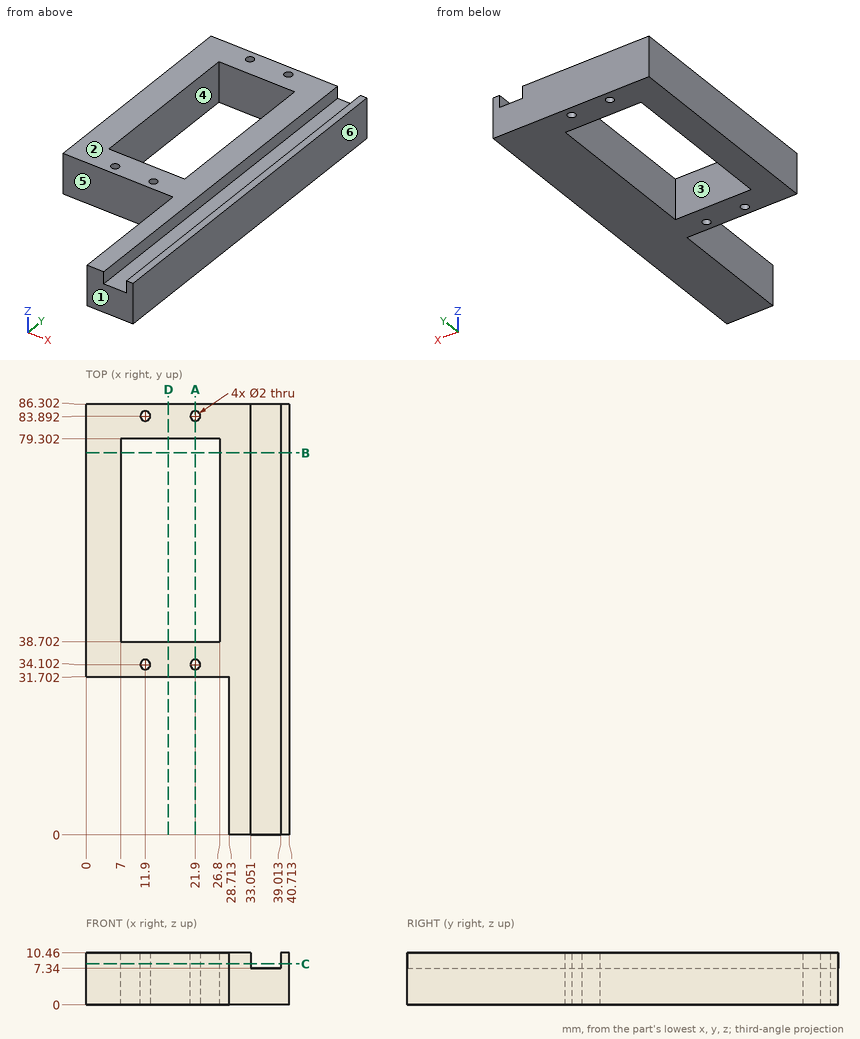
Design review of the part shown in the three views and the two pictorial views. Dimensions are in mm from the part's minimum x, y and z. A direction names the side the tool comes from. Give positions to 0.01 mm unless a question says otherwise; leave off trailing zeros. Loops run counter-clockwise (first coordinate to the right, second up) from the corner with the lowest first, then second, coordinate; pieces in that order, holes last. Notation, with made-up numbers: (34, 62.25) -> (64, 62.25) arc R30 cw to (64, 91.25) -> close; hole circle Ø9 at (51.25, -26.5). An arc over 180 degrees is marked (long way). Answer as a JSON object with one key per item and string values. Group by question number.
Q1. Draft analysis for pull direction Y (two halves, no side actions). For the marked faces 1, 2 and 3, state which applies: pulls with the +Y half, pulls with the -Y half, needs draft (parallel to the pull), parting line crosses it, or undercut.
Q2. Wall thickness on line 1 along Y through (x, z) = (11.9, 4); line 2 along X through (y, z) = (58, 8.75); line 3 along Y through (x, z) = (24, 9.75): over which ranges is each line inside the solid? List them lowest first.
Q3. Tool access review of the marked faces 4, 5 and 6: name each direction out of +Z, -Z, +X, -X, +Y, -Y from which nothing blocks a thin tool from reaching the whole face with its end or side.
Q4. Insertion check: pin 1 (3 mm diameter, centred on x = 21.9, y = 83.89, fed in from -Z); pin 2 (0.9 mm diameter, centred on y = 28, z = 9.5, fed in from -X); pin 3 (1.8 mm diameter, centred on x = 36.5, y = 50.5, fed in from +Z); pin 4 (3 mm diameter, centred on x = 21, z = 2.5, fed in from -Y). Each pin has a flat end and moves straight along its axis. Give the tip position at first contact, or say it passes through.
Q5. Take a section at A-A (x = 21.9). Write out the cut boundary in (y, z).
Q6. Take a section at D-D (x = 16.5). Write out the cut boundary in (y, z), plus the area to 3 significant figures.
Q7. Take a section at B-B (y = 76.5). Write out the cut boundary in (x, z), plus the area to 3 significant figures.
Q8. Take a section at C-C (z = 8.25). Write out the cut boundary in (x, y), plus the area to 3 significant figures.
Answer below:
{
 "1": {"face 1": "pulls with the -Y half", "face 2": "needs draft", "face 3": "undercut"},
 "2": {"line 1": "y = 31.7 to 33.1, 35.1 to 38.7, 79.3 to 82.89, 84.89 to 86.3", "line 2": "x = 0 to 7, 26.8 to 33.05, 39.01 to 40.71", "line 3": "y = 31.7 to 38.7, 79.3 to 86.3"},
 "3": {"face 4": "+Z, -Z", "face 5": "+Z, -Z, -X, -Y", "face 6": "+Z, -Z, +X, +Y, -Y"},
 "4": {"pin 1": "stops at z = 0", "pin 2": "stops at x = 28.71", "pin 3": "stops at z = 7.34", "pin 4": "stops at y = 31.7"},
 "5": {"outline": "(31.7, 0) -> (33.1, 0) -> (33.1, 10.46) -> (31.7, 10.46) -> close; (35.1, 0) -> (38.7, 0) -> (38.7, 10.46) -> (35.1, 10.46) -> close; (79.3, 0) -> (82.89, 0) -> (82.89, 10.46) -> (79.3, 10.46) -> close; (84.89, 0) -> (86.3, 0) -> (86.3, 10.46) -> (84.89, 10.46) -> close"},
 "6": {"outline": "(31.7, 0) -> (38.7, 0) -> (38.7, 10.46) -> (31.7, 10.46) -> close; (79.3, 0) -> (86.3, 0) -> (86.3, 10.46) -> (79.3, 10.46) -> close", "area": "146 mm2"},
 "7": {"outline": "(0, 0) -> (7, 0) -> (7, 10.46) -> (0, 10.46) -> close; (26.8, 0) -> (40.71, 0) -> (40.71, 10.46) -> (39.01, 10.46) -> (39.01, 7.34) -> (33.05, 7.34) -> (33.05, 10.46) -> (26.8, 10.46) -> close", "area": "200 mm2"},
 "8": {"outline": "(0, 31.7) -> (28.71, 31.7) -> (28.71, 0) -> (33.05, 0) -> (33.05, 86.3) -> (0, 86.3) -> close; (39.01, 0) -> (40.71, 0) -> (40.71, 86.3) -> (39.01, 86.3) -> close; hole (7, 38.7) -> (26.8, 38.7) -> (26.8, 79.3) -> (7, 79.3) -> close; hole circle Ø2 at (11.9, 34.1); hole circle Ø2 at (11.9, 83.89); hole circle Ø2 at (21.9, 34.1); hole circle Ø2 at (21.9, 83.89)", "area": "1,270 mm2"}
}
